Job drawing, mm, ordinate dimensions from the low corner. One solid piece. Give positions to 0.01 mm unless a question says otherwise; leave off trailing zeros. Loops run counter-clockwise (first coordinate to the right, second up) from the corner with the lowest first, then second, coordinate; pieces in that order, holes last. Notation, with made-up numbers: M 79.5,-31.5 L 110.5,-31.5 A10 ccw 110.5,-14.5 Z; hole C 5,5.5 d7. An arc over 180 degrees is marked long. Put each result on its own line as item: value.
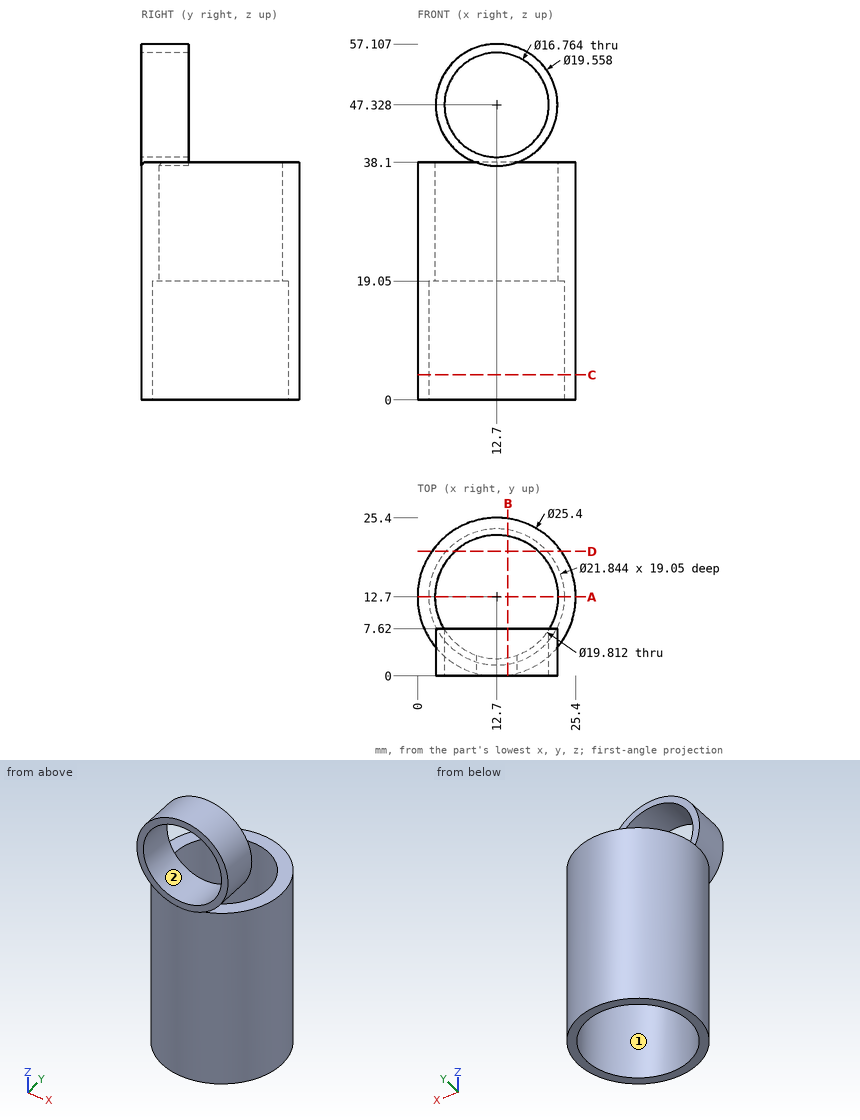
Q1. Drop flat-ended pins along their axis: pin 1 Ø8 at (y, z) = (7, 32) entering from +X; pin 2 Ø4 at (y, z) = (19.5, 21) entering from -X; pin 3 Ø10 at (x, y) = (10, 21) entering from +Z; pin 4 Ø7.5 at (x, y) = (14.5, 17.5) entering from +Z. Give the stop position or say it passes through.
Here are the results:
pin 1: x = 25.29
pin 2: x = 0.94
pin 3: z = 38.1
pin 4: through
Q2. Slice it at D-D (y = 20). List the corners of the cut face in (x, z).
Here are the results:
outline: M 2.31,0 L 4.58,0 L 4.58,19.05 L 6,19.05 L 6,38.1 L 2.31,38.1 Z; M 19.4,19.05 L 20.82,19.05 L 20.82,0 L 23.09,0 L 23.09,38.1 L 19.4,38.1 Z
Q3. Mould opens along Z. For the marked faces 1 and 2 say: pulls with the +Z half, pulls with the -Z half, needs draft (parallel to the pull), parting line crosses it, or undercut.
Here are the results:
face 1: needs draft
face 2: undercut
Q4. Slice it at B-B (x = 14.5). List the corners of the cut face in (y, z).
Here are the results:
outline: M 0,37.72 L 0.13,37.72 L 0.13,0 L 1.93,0 L 1.93,19.05 L 2.96,19.05 L 2.96,37.72 L 7.62,37.72 L 7.62,39.14 L 0,39.14 Z; M 0,55.51 L 7.62,55.51 L 7.62,56.94 L 0,56.94 Z; M 22.44,19.05 L 23.47,19.05 L 23.47,0 L 25.27,0 L 25.27,38.1 L 22.44,38.1 Z
Q5. Probe line 1 (Z direction, x = 12.7, y = 5); line 2 (Y direction, x = 12.7, z = 12); line 3 (Y direction, x = 12.7, z = 30.25). List the from-to ranges inside material, lowest first. Write a range as from..to.
Here are the results:
line 1: 37.55..38.95, 55.71..57.11
line 2: 0..1.78, 23.62..25.4
line 3: 0..2.79, 22.61..25.4
Q6. Slice it at A-A (y = 12.7). List the corners of the cut face in (x, z), and give its area (3 significant figures).
Here are the results:
outline: M 0,0 L 1.78,0 L 1.78,19.05 L 2.79,19.05 L 2.79,38.1 L 0,38.1 Z; M 22.61,19.05 L 23.62,19.05 L 23.62,0 L 25.4,0 L 25.4,38.1 L 22.61,38.1 Z
area: 174 mm²
Q7. Slice it at C-C (z = 4). List the corners of the cut face in (x, y).
Here are the results:
outline: C 12.7,12.7 d25.4; hole C 12.7,12.7 d21.84
